The drawing under review shows one solid part. Ordinate dimensions are in mm from its lowest x, y, z. A direction names the side the tool comes from. Give positions to 0.01 mm unless a question says otherwise; leave off trailing zeros. Write each loop counter-clockwise with the first axis right and the second up, starting at its lowest first coordinate (ties: lowest second). Pieces come first, ordered by that corner, then holes. Notation, with made-up numbers: (-13.75, -26) -> (24.25, -26) arc R16 ccw to (24.25, -2) -> close; hole circle Ø9 at (63, 59). An arc over 180 degrees is marked (long way). Answer as a JSON object with one key per item and string values.
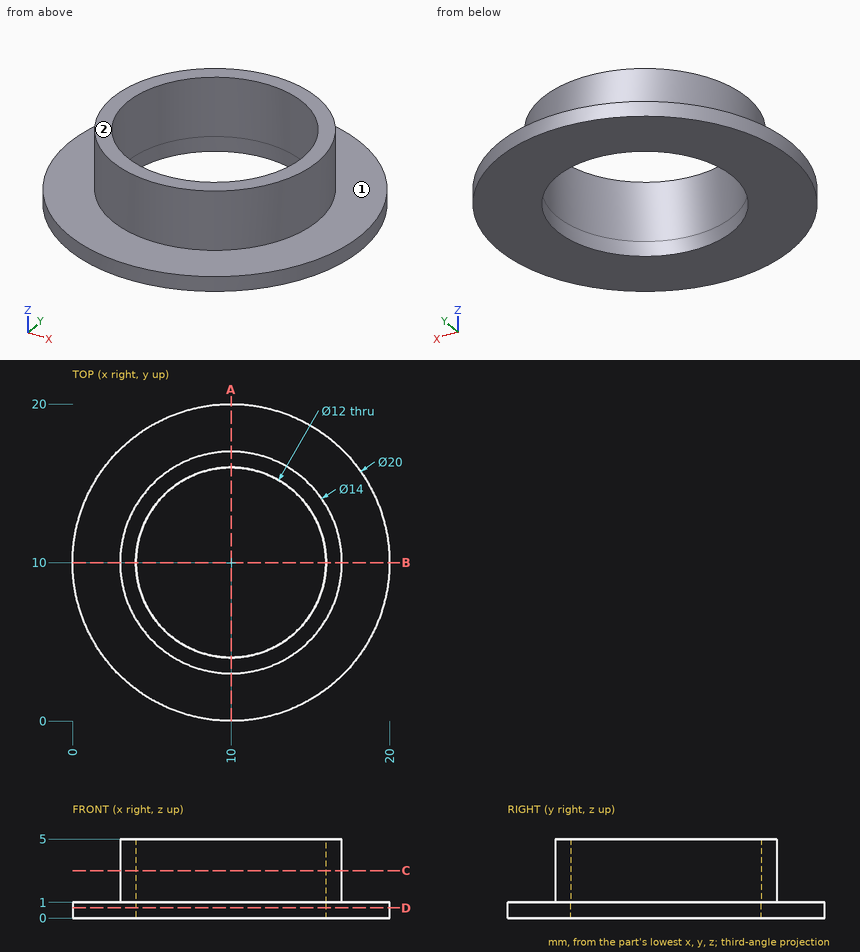
(1) Clearance check with flat-ended pins moving along their axes: pin 1 (1.5 mm diameter, centred on x = 9.5, y = 13.5, fed in from +Z); pin 2 (1 mm diameter, centred on y = 13.5, z = 3.5, fed in from +X). State where each tip first meets the part, or that it passes through.
Here are the results:
{"pin 1": "passes through", "pin 2": "stops at x = 16.32"}
(2) We need section A-A, the plane x = 10. State the section outline as (y, z) points.
Here are the results:
{"outline": "(0, 0) -> (4, 0) -> (4, 5) -> (3, 5) -> (3, 1) -> (0, 1) -> close; (16, 0) -> (20, 0) -> (20, 1) -> (17, 1) -> (17, 5) -> (16, 5) -> close"}
(3) For line 1 along Y through (x, z) = (10, 0.25); line 2 along X through (y, z) = (10.25, 0.75); line 3 along Y through (x, z) = (10, 4), list the stretches that pass through material, from the lowest coordinate up.
Here are the results:
{"line 1": "y = 0 to 4, 16 to 20", "line 2": "x = 0 to 4.01, 15.99 to 20", "line 3": "y = 3 to 4, 16 to 17"}
(4) We need section D-D, the plane z = 0.65. State the section outline as (x, y) points.
Here are the results:
{"outline": "circle Ø20 at (10, 10); hole circle Ø12 at (10, 10)"}
(5) We need section C-C, the plane z = 3. State the section outline as (x, y) points.
Here are the results:
{"outline": "circle Ø14 at (10, 10); hole circle Ø12 at (10, 10)"}
(6) For the marked faces 1 and 2, list the 3-axis set-ups (+Z, -Z, +X, -X, +Y, -Y) from which the entire face can be reached by the end or side of a thin tool; tool diameter is ignored.
Here are the results:
{"face 1": "+Z", "face 2": "+Z, +X, -X, +Y, -Y"}
